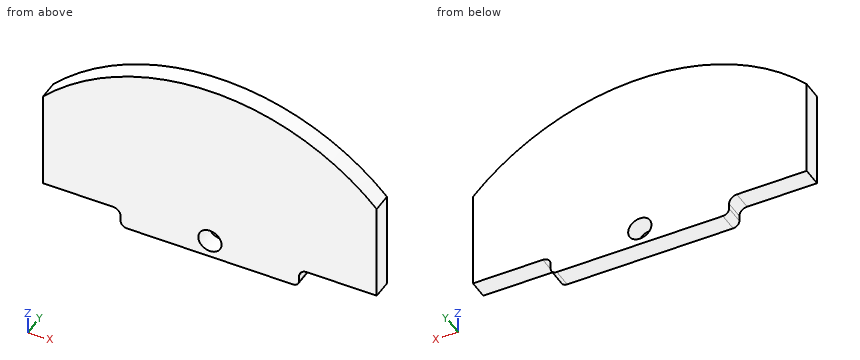
```python
from build123d import *

# Parameters (mm, degrees)
BOSS_EXTRUDE2_DEPTH = 6.35
SKETCH10_W          = 25.4
SKETCH10_H          = 6.35
CUT_EXTRUDE1_DEPTH  = 7.35
FILLET1_R           = 2.54
FILLET2_R           = 2.032
SKETCH11_R          = 3.81
CUT_EXTRUDE2_DEPTH  = 7.35


with BuildPart() as part:
    # Sketch6 → Boss-Extrude2 (new body)
    with BuildSketch(Plane(origin=(0, 0, 0), x_dir=(1, 0, 0), z_dir=(0, 1, 0))):
        with BuildLine():
            Line((0, 0), (109.1946, 0))
            Line((109.1946, 0), (109.1946, -38.862))
            ThreePointArc((109.1946, -38.862), (54.5973, -61.992965275), (0, -38.862))
            Line((0, -38.862), (0, 0))
        make_face()
    extrude(amount=BOSS_EXTRUDE2_DEPTH)

    # Sketch10 → Cut-Extrude1 (cut, through all)
    with BuildSketch(Plane(origin=(0, 6.35, 0), x_dir=(1, 0, 0), z_dir=(0, 1, 0))):
        with Locations((96.4946, -3.175)):
            Rectangle(SKETCH10_W, SKETCH10_H)
        with Locations((12.7, -3.175)):
            Rectangle(SKETCH10_W, SKETCH10_H)
    extrude(amount=-CUT_EXTRUDE1_DEPTH, mode=Mode.SUBTRACT)

    # Fillet1
    fillet1_edges = [part.edges().sort_by_distance(p)[0] for p in [
        (25.4, 3.175, 6.35),
        (83.7946, 3.175, 6.35),
    ]]
    fillet(fillet1_edges, radius=FILLET1_R)

    # Fillet2
    fillet2_edges = [part.edges().sort_by_distance(p)[0] for p in [
        (25.4, 3.175, 0),
        (83.7946, 3.175, 0),
    ]]
    fillet(fillet2_edges, radius=FILLET2_R)

    # Sketch11 → Cut-Extrude2 (cut, through all)
    with BuildSketch(Plane.XZ):
        with Locations((54.61, 5.819375203)):
            Circle(SKETCH11_R)
    extrude(amount=-CUT_EXTRUDE2_DEPTH, mode=Mode.SUBTRACT)


solid = part.part
```
Check sheet for the modelled part. Datum: model origin and axes. Units: mm. Round coordinates to 2 decimals unless told otherwise and drop trailing zeros. Loops run counter-clockwise (first coordinate to the right, second up) from the corner with the lowest first, then second, coordinate; pieces in that order, holes last. Notation, with made-up numbers: (14.25, -2) - (59.25, -2) arc R19 ccw to (59.25, 11) - close; hole circle Ø2 at (47, 32.25). An arc over 180 degrees is marked (long way). Answer as a JSON object with one key per item and string values. Group by question number.
Q1. Sectioned sample at A-A, the plane x = 54.61. Enter the section's corners in (y, z), plus the area to 3 significant figures.
Q2. Scan lines: line 1 along Z through (x, y) = (54.61, 2.5); line 2 along Z through (x, y) = (42, 6.25); line 3 along X through (y, z) = (4.75, 40). Record each from-to range of solid material in increasing order. Write a range as [from, to].
Q3. Sectioned sample at C-C, the plane z = 48.5. Enter the section's corners in (x, y), plus the area to 3 significant figures.
Q4. Sectioned sample at B-B, the plane y = 2.75. Enter the section's corners in (x, z).
Q5. Gauge pin test, flat ends, axial feed: P1, Ø0.5, axis at y = 3.5, z = 2.5, coming from the +X side; P2, Ø3, axis at x = 17, y = 5, coming from the +Z side; P3, Ø1.4, axis at y = 4.5, z = 3, coming from the -X side. Record the tip position at first contact, or that the pin passes through.
Q6. Sectioned sample at D-D, the plane x = 98.5. Enter the section's corners in (y, z), plus the area to 3 significant figures.
Solution:
{
 "1": {"outline": "(0, 0) - (6.35, 0) - (6.35, 2.01) - (0, 2.01) - close; (0, 9.63) - (6.35, 9.63) - (6.35, 61.99) - (0, 61.99) - close", "area": "345 mm²"},
 "2": {"line 1": "z = [0, 2.01], [9.63, 61.99]", "line 2": "z = [0, 60.94]", "line 3": "x = [1.13, 108.07]"},
 "3": {"outline": "(11.37, 0) - (97.83, 0) - (97.83, 6.35) - (11.37, 6.35) - close", "area": "549 mm²"},
 "4": {"outline": "(0, 6.35) - (22.86, 6.35) arc R2.54 cw to (25.4, 3.81) - (25.4, 2.03) arc R2.03 ccw to (27.43, 0) - (81.76, 0) arc R2.03 ccw to (83.79, 2.03) - (83.79, 3.81) arc R2.54 cw to (86.33, 6.35) - (109.19, 6.35) - (109.19, 38.86) arc R76 ccw to (0, 38.86) - close; hole circle Ø7.62 at (54.61, 5.82)"},
 "5": {"P1": "stops at x = 83.79", "P2": "stops at z = 52.87", "P3": "stops at x = 25.4"},
 "6": {"outline": "(0, 6.35) - (6.35, 6.35) - (6.35, 48.03) - (0, 48.03) - close", "area": "265 mm²"}
}
